Part model, mm, in its own coordinate system. Face numbers are marked on the shaded views. Give positions to 0.01 mm unless a question says otherwise; leave off trailing zeros. Order: outer loops, then holes, each group sorted by start corner. A loop starts at its lowest first (then second) coordinate and runs counter-clockwise, first axis right, second up. Notation, with made-up numbers: (81, -17) -> (113, -17) arc R16 ccw to (113, 5) -> close; hole circle Ø8 at (37, 46). An arc over 180 degrees is marked (long way). Write item = value, one per line. Start each with the question number.
Item 1: Flat gauge pins, fed straight in: P1, Ø6, axis at y = -2.5, z = 14, coming from the +X side; P2, Ø7, axis at y = 0, z = 18.4, coming from the +X side; P3, Ø4, axis at y = -7.5, z = 2, coming from the +X side. Where does each tip first touch, or does it go through?
Item 2: Band-saw the part on A-A on z = 8.4. Write the cut outline in (x, y).
Item 3: Band-saw the part on D-D on x = 25. Write the cut outline in (y, z).
Item 4: Band-saw the part on C-C on y = 0. Write the cut outline in (x, z).
Item 5: Pull direction Y, two halves, no side cores. Call the marked faces 1, 2 and 3: +Y half, -Y half, draft (parallel to the pull), parting line (faces both ways), or undercut.
Item 6: Band-saw the part on B-B on x = 12. Write the cut outline in (y, z), plus the area to 3 significant figures.
Item 7: Drill centre lines: line 1 along Z through (x, y) = (13, 0); line 2 along Y through (x, z) = (10, 8.4); line 3 along Y through (x, z) = (6, 18.4). Where is each one in solid material? Low to high.
Autodesk Inventor part; units mm, degrees
ref_plane "YZ Plane" through (0, 0, 0) normal (1, 0, 0) x (0, 1, 0)
ref_plane "XZ Plane" through (0, 0, 0) normal (0, 1, 0) x (-1, 0, 0)
ref_plane "XY Plane" through (0, 0, 0) normal (0, 0, 1) x (1, 0, 0)
sketch "Sketch1" plane through (0, 0, 0) normal (0, 0, 1) x (1, 0, 0)
  line L0 (0, -25.4) -> (33.233, -25.4)
  line L1 (33.233, 25.4) -> (0, 25.4)
  line L2 (0, 25.4) -> (0, -25.4)
  circle A0 centre (49.5, 0) radius 30.1625 construction
  line L3 (0, 0) -> (-12.014, 0)
  arc A1 (33.233, 25.4) -> (33.233, -25.4) centre (49.5, 0) ccw
  point P0 (0, 0)
  dimension "d0" = 60.325
  dimension "d1" = 49.5
  dimension "d2" = 50.8
extrude "Extrusion1" add sketch "Sketch1" along normal mid plane 50.8
sketch "Sketch2" plane through (0, -25.4, 25.4) normal (-1, 0, 0) x (0, 0, 1)
  circle A0 centre (-7, 25.4) radius 2.75
  circle A1 centre (-17, 25.4) radius 2.75
  line L0 (0, 50.8) -> (0, 0)
  point P0 (-25.4, 25.4)
  dimension "d8" = 5.5
  dimension "d9" = 7
  dimension "d10" = 10
extrude "Extrusion2" cut sketch "Sketch2" against normal through all
fillet "Fillet1" radius 10 4 edges at (16.6165, 25.4, 25.4) (16.6165, -25.4, 25.4) (16.6165, 25.4, -25.4) (16.6165, -25.4, -25.4)
properties part number "Pipe Holder" material "ABS Plastic"
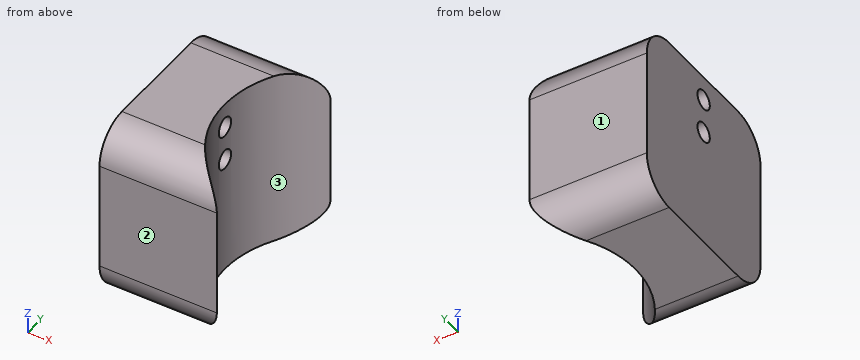
Values found:
q1.P1 = 19.84
q1.P2 = 19.54
q1.P3 = 20.87
q2.outline = (0, -25.4) -> (33.23, -25.4) arc R30.16 cw to (19.46, -2.75) -> (0, -2.75) -> close; (0, 2.75) -> (19.46, 2.75) arc R30.16 cw to (33.23, 25.4) -> (0, 25.4) -> close
q3.outline = (-25.4, -15.4) arc R10 ccw to (-17.59, -25.16) -> (-17.59, 25.16) arc R10 ccw to (-25.4, 15.4) -> close; (17.59, -25.16) arc R10 ccw to (25.4, -15.4) -> (25.4, 15.4) arc R10 ccw to (17.59, 25.16) -> close
q4.outline = (0, -25.4) -> (19.34, -25.4) -> (19.34, 5.65) -> (0, 5.65) -> close; (0, 11.15) -> (19.34, 11.15) -> (19.34, 15.65) -> (0, 15.65) -> close; (0, 21.15) -> (19.34, 21.15) -> (19.34, 25.4) -> (0, 25.4) -> close
q5.face_1 = +Y half
q5.face_2 = -Y half
q5.face_3 = undercut
q6.outline = (-25.4, -15.4) arc R10 ccw to (-15.4, -25.4) -> (15.4, -25.4) arc R10 ccw to (25.4, -15.4) -> (25.4, 15.4) arc R10 ccw to (15.4, 25.4) -> (-15.4, 25.4) arc R10 ccw to (-25.4, 15.4) -> close; hole circle Ø5.5 at (0, 8.4); hole circle Ø5.5 at (0, 18.4)
q6.area = 2,450 mm^2
q7.line_1 = -25.4 to 5.65, 11.15 to 15.65, 21.15 to 25.4
q7.line_2 = -25.4 to -2.75, 2.75 to 25.4
q7.line_3 = -24.94 to -2.75, 2.75 to 24.94
